Geometry: final body of the model. Coordinates: model frame, mm. A direction names the side the tool comes from. Give positions to 0.01 mm unless a question says otherwise; leave off trailing zeros. Write each loop counter-clockwise with the first axis right and the second up, starting at its lowest first coordinate (ties: lowest second). Pieces come first, ordered by that corner, then holes.
Q1. Reachability of faces 4 (the face through (-217.169, 17, 3)), 5 (the face through (-251, -35.204, 15)), 6 (the face through (-177.669, 24, 20)) from +Z, -Z, +X, -X, +Y, -Y: full face, straight path, thin tool, end or side. Return the list, or none.
Q2. Pin query (flat end, axial travel): pin 1 (10 mm diameter, centred on x = -207, y = 33, fed in from +Z); pin 2 (7 mm diameter, centred on x = -290, z = 4, fed in from -Y); pin 3 (2 mm diameter, centred on x = -208.5, z = 2.5, fed in from -Y); pin 4 (6 mm diameter, centred on x = -294.67, y = 49.8, fed in from -Z). Return the tip coordinate at first contact, or that it passes through.
Q3. Cut plane D-D on y = 7. Return the cut outline in (x, z).
Q4. Cut plane A-A on x = -199.5. Return the cut outline in (y, z).
Q5. Cut plane B-B on z = 17. Return the cut outline in (x, y).
Q6. Line query: L1, parallel to X at y = -4.5, z = 6.25; L2, parallel to Y at x = -198.5, z = 12.75; L3, parallel to Y at x = -241, z = 7.75. Output: solid intervals per line, ascending.
Q7. Draft query along Y for faces 1 (the face through (-294, 18, 6.5)), 2 (the face through (-204, 69.796, 3)), 3 (the face through (-202.36, -16.16, 8.27)). Return one class per face: pulls with the +Y half, pulls with the -Y half, needs draft (parallel to the pull), parting line crosses it, or undercut.
Q8. Cut plane C-C on x = -271. Return the cut outline in (y, z), plus the area to 3 significant figures.
```python
from build123d import *

# Parameters (mm, degrees)
SKETCH1_W                 = 150
SKETCH1_H                 = 120
BOSS_EXTRUDE1_DEPTH       = 30
SKETCH2_W                 = 25
SKETCH2_H                 = 105
CUT_EXTRUDE1_DEPTH        = 6.5
SKETCH4_W                 = 144
SKETCH4_H                 = 114
CUT_EXTRUDE2_DEPTH        = 20
FILLET1_R                 = 10
F_5_0MM_DOWEL_HOLE1_D     = 5
F_5_0MM_DOWEL_HOLE1_DEPTH = 20
F_5_0MM_DOWEL_HOLE1_TIP   = 1.502151548
SKETCH12_W                = 50
SKETCH12_H                = 10
CUT_EXTRUDE6_DEPTH        = 337.897861193


with BuildPart() as part:
    # Sketch1 → Boss-Extrude1 (new body)
    with BuildSketch(Plane.XY):
        with Locations((-249.668715257, 24.796192189)):
            Rectangle(SKETCH1_W, SKETCH1_H)
    extrude(amount=BOSS_EXTRUDE1_DEPTH)

    # Sketch2 → Cut-Extrude1 (cut)
    with BuildSketch(Plane(origin=(0, 0, 0), x_dir=(-1, 0, 0), z_dir=(0, 0, -1))):
        with Locations((204.668715257, 17.296192189)):
            Rectangle(SKETCH2_W, SKETCH2_H)
        with Locations((294.668715257, 17.296192189)):
            Rectangle(SKETCH2_W, SKETCH2_H)
    extrude(amount=-CUT_EXTRUDE1_DEPTH, mode=Mode.SUBTRACT)

    # Sketch4 → Cut-Extrude2 (cut)
    with BuildSketch(Plane.XY.offset(30)):
        with Locations((-249.668715257, 24.796192189)):
            Rectangle(SKETCH4_W, SKETCH4_H)
    extrude(amount=-CUT_EXTRUDE2_DEPTH, mode=Mode.SUBTRACT)

    # Fillet1
    fillet1_edges = [part.edges().sort_by_distance(p)[0] for p in [
        (-177.668715257, 81.796192189, 20),
        (-177.668715257, -32.203807811, 20),
        (-321.668715257, -32.203807811, 20),
        (-321.668715257, 81.796192189, 20),
        (-174.668715257, -35.203807811, 15),
        (-324.668715257, -35.203807811, 15),
        (-324.668715257, 84.796192189, 15),
        (-174.668715257, 84.796192189, 15),
    ]]
    fillet(fillet1_edges, radius=FILLET1_R)

    # Ø5.0mm Dowel Hole1
    with Locations(Plane(origin=(0, 0, 6.5), x_dir=(-1, 0, 0), z_dir=(0, 0, -1))):
        with Locations((204.668715257, 49.796192189), (204.668715257, -15.203807811), (294.668715257, 49.796192189), (294.668715257, -15.203807811)):
            Hole(F_5_0MM_DOWEL_HOLE1_D / 2, depth=F_5_0MM_DOWEL_HOLE1_DEPTH)
            with Locations((0, 0, -(F_5_0MM_DOWEL_HOLE1_DEPTH + F_5_0MM_DOWEL_HOLE1_TIP / 2))):  # 118° drill point
                Cone(0, F_5_0MM_DOWEL_HOLE1_D / 2, F_5_0MM_DOWEL_HOLE1_TIP, mode=Mode.SUBTRACT)

    # Sketch12 → Cut-Extrude6 (cut, through all)
    with BuildSketch(Plane(origin=(0, 0, 0), x_dir=(-1, 0, 0), z_dir=(0, 0, -1))):
        with Locations((249.668715257, -10.203807811)):
            Rectangle(SKETCH12_W, SKETCH12_H)
    extrude(amount=-CUT_EXTRUDE6_DEPTH, mode=Mode.SUBTRACT)


solid = part.part
```
Data:
1. face 4: -Z, -Y
1. face 5: +Z, -Z, +X, -X, -Y
1. face 6: +Z
2. pin 1: stops at z = 10
2. pin 2: stops at y = -35.2
2. pin 3: stops at y = 69.8
2. pin 4: stops at z = 6.5
3. outline: (-324.67, 0) - (-307.17, 0) - (-307.17, 6.5) - (-282.17, 6.5) - (-282.17, 0) - (-217.17, 0) - (-217.17, 6.5) - (-192.17, 6.5) - (-192.17, 0) - (-174.67, 0) - (-174.67, 30) - (-177.67, 30) - (-177.67, 10) - (-321.67, 10) - (-321.67, 30) - (-324.67, 30) - close
4. outline: (-35.2, 6.5) - (69.8, 6.5) - (69.8, 0) - (84.8, 0) - (84.8, 30) - (81.8, 30) - (81.8, 10) - (-32.2, 10) - (-32.2, 30) - (-35.2, 30) - close
5. outline: (-324.67, -25.2) arc R10 ccw to (-314.67, -35.2) - (-184.67, -35.2) arc R10 ccw to (-174.67, -25.2) - (-174.67, 74.8) arc R10 ccw to (-184.67, 84.8) - (-314.67, 84.8) arc R10 ccw to (-324.67, 74.8) - close; hole (-321.67, -22.2) arc R10 ccw to (-311.67, -32.2) - (-187.67, -32.2) arc R10 ccw to (-177.67, -22.2) - (-177.67, 71.8) arc R10 ccw to (-187.67, 81.8) - (-311.67, 81.8) arc R10 ccw to (-321.67, 71.8) - close
6. L1: x = -324.67 to -307.17, -282.17 to -217.17, -192.17 to -174.67
6. L2: y = -35.2 to -32.2, 81.8 to 84.8
6. L3: y = -35.2 to -15.2, -5.2 to 84.8
7. face 1: needs draft
7. face 2: pulls with the -Y half
7. face 3: undercut
8. outline: (-35.2, 0) - (-15.2, 0) - (-15.2, 10) - (-32.2, 10) - (-32.2, 30) - (-35.2, 30) - close; (-5.2, 0) - (84.8, 0) - (84.8, 30) - (81.8, 30) - (81.8, 10) - (-5.2, 10) - close
8. area: 1,220 mm2
